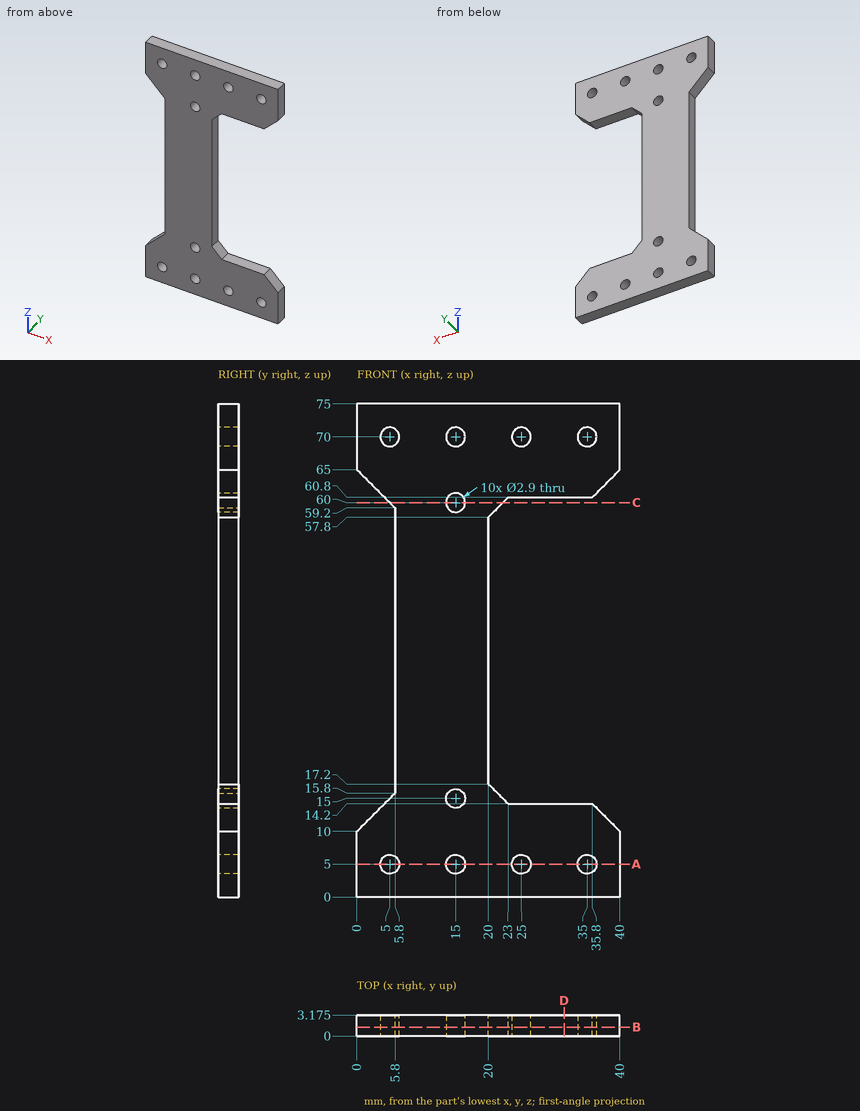
Geometry check sheet. Reference: drawing and pictorial views, mm from the part's lowest x, y, z. Give positions to 0.01 mm unless a question says otherwise; leave off trailing zeros. Write each loop counter-clockwise with the first axis right and the second up, starting at its lowest first coordinate (ties: lowest second). Pieces come first, ordered by that corner, then holes. Notation, with made-up numbers: M -16.5,-20.75 L 26.5,-20.75 A24 cw 26.5,15.25 Z; hole C -20.5,-14.5 d2. An arc over 180 degrees is marked long. Answer as CSV lines item,"result". Start each with the question number.
Q1. Material ranges on L1, parallel to X at y = 1.9, z = 70; L2, parallel to Z at x = 15, y = 0.7; L3, parallel to Z at x = 5, y = 1.55, recorded low to high.
Q2. Section check B-B, the plane y = 1.35. Give the number of separate pieces and of enclosed holes in the cut face, then the cut area to 3 significant figures.
Q3. Section check A-A, the plane z = 5. Record the cut outline in (x, y) (3 decimals), then the cut area to 3 significant figures.
Q4. Go/stop test with flat-tipped pins: pin 1 (4.5 mm diameter, centred on x = 15, z = 70, fed in from +Y) (3 decimals); pin 2 (2.5 mm diameter, centred on x = 35, z = 5, fed in from +Y); pin 3 (1 mm diameter, centred on y = 1.5, z = 38, fed in from -X); pin 4 (1 mm diameter, centred on y = 2, z = 42.5, fed in from +X). Record where each tip stops, or that it passes through.
Q5. Section check D-D, the plane x = 31.5. Record the cut outline in (y, z) (3 decimals).
Q6. Section check C-C, the plane z = 60. Record the cut outline in (x, y) (3 decimals), then the cut area to 3 significant figures.
Geometry says:
1,L1,"0 to 3.55, 6.45 to 13.55, 16.45 to 23.55, 26.45 to 33.55, 36.45 to 40"
1,L2,"0 to 3.55, 6.45 to 13.55, 16.45 to 58.55, 61.45 to 68.55, 71.45 to 75"
1,L3,"0 to 3.55, 6.45 to 15, 60 to 68.55, 71.45 to 75"
2,separate pieces,"1"
2,enclosed holes,"10"
2,area,"1,710 mm^2"
3,outline,"M 0,0 L 3.55,0 L 3.55,3.175 L 0,3.175 Z; M 6.45,0 L 13.55,0 L 13.55,3.175 L 6.45,3.175 Z; M 16.45,0 L 23.55,0 L 23.55,3.175 L 16.45,3.175 Z; M 26.45,0 L 33.55,0 L 33.55,3.175 L 26.45,3.175 Z; M 36.45,0 L 40,0 L 40,3.175 L 36.45,3.175 Z"
3,area,"90.2 mm^2"
4,pin 1,"y = 3.175"
4,pin 2,"through"
4,pin 3,"x = 5.8"
4,pin 4,"x = 20"
5,outline,"M 0,0 L 3.175,0 L 3.175,14.2 L 0,14.2 Z; M 0,60.8 L 3.175,60.8 L 3.175,75 L 0,75 Z"
6,outline,"M 5,0 L 13.55,0 L 13.55,3.175 L 5,3.175 Z; M 16.45,0 L 22.2,0 L 22.2,3.175 L 16.45,3.175 Z"
6,area,"45.4 mm^2"
